Here's how the part is built. I have some questions about the finished solid (model axes, mm). A direction names the side the tool comes from. Round coordinates to 2 decimals unless told otherwise and drop trailing zeros. Order: outer loops, then holes, each group sorted by start corner. A loop starts at its lowest first (then second) coordinate and runs counter-clockwise, first axis right, second up. Notation, with made-up numbers: M -4,69.5 L 41,69.5 A20 cw 41,80.5 Z; hole C -18.5,1 d8. An arc over 180 degrees is marked long. Write item = value, one per line. Start each with the question number.
Item 1: I want a section at A-A, the plane x = 126.5. List the corners of the cut face in (y, z) for me.
Item 2: I want a section at B-B, the plane z = 3.75. State how many separate pieces and enclosed holes the cut face has, plus the area to 3 significant figures.
Item 3: I want a section at C-C, the plane x = -10. List the corners of the cut face in (y, z) for me.
Item 4: Please list where these lines run through material, in increasing order: L1, parallel to Y at x = 111, z = 3.25; L2, parallel to Y at x = 91.5, z = 6.5; L3, parallel to Y at x = 125, z = 6.
Item 5: I'm going to push flat-ended pins straight in: P1, Ø5.5, axis at x = 142.21, y = 21.4, coming from the +Z side; P2, Ø2, axis at x = -7.5, z = 6, coming from the +Y side; P3, Ø0.6, axis at y = 32.5, z = 4, coming from the +X side; P4, Ø1.4, axis at y = 17, z = 3.5, coming from the -X side. Where does each tip first touch, or does it pass through?
Item 6: For faces 1 (the face through (63.856, 15, 4)), 2 (the face through (131.856, 17, 4)), 3 (the face through (137.856, 21, 4)), 4 (the face through (134.9, 26.11, 4.37)), which set-ups out of +Z, -Z, +X, -X, +Y, -Y let a thin tool reach every point of the face, with its end or its side?
```python
from build123d import *

# Parameters (mm, degrees)
F1_DEPTH = 6.8
F2_T     = -2
F4_DEPTH = 4.8
F6_DEPTH = 4.8
F5_R     = 3.15
F7_DEPTH = 2


# Not quite as in the source:
# - a feature names something its author has since deleted; it is built from what else it names


with BuildPart() as f1:
    # F0 (on Top) → F1 (new body)
    with BuildSketch(Plane.XY):
        with BuildLine():
            Line((129.8559711718, 33.7323809788), (-4.1440288282, 33.7323809788))
            ThreePointArc((-4.1440288282, 33.7323809788), (-21.8216983579, 26.4100505084), (-29.1440288282, 8.7323809788))
            Line((-29.1440288282, 8.7323809788), (154.8559711718, 8.7323809788))
            ThreePointArc((154.8559711718, 8.7323809788), (147.5336407015, 26.4100505084), (129.8559711718, 33.7323809788))
        make_face()
    extrude(amount=F1_DEPTH)

    # F2
    f2_openings = [f1.faces().sort_by_distance(p)[0] for p in [
        (62.855971, 20.804106, 6.8),
    ]]
    offset(amount=F2_T, openings=f2_openings)

    # F3 (on face) → F4 (cut)
    with BuildSketch(Plane.XY.offset(6.8)):
        with BuildLine():
            Line((-4.1440288282, 8.7323809788), (-4.1440288282, 10.7323809788))
            Line((-4.1440288282, 10.7323809788), (-27.056907303, 10.7323809788))
            ThreePointArc((-27.056907303, 10.7323809788), (-19.6842990961, 25.6882059366), (-4.1440288282, 31.7323809788))
            Line((-4.1440288282, 31.7323809788), (-4.1440288282, 33.7323809788))
            ThreePointArc((-4.1440288282, 33.7323809788), (-21.8216983579, 26.4100505084), (-29.1440288282, 8.7323809788))
            Line((-29.1440288282, 8.7323809788), (-4.1440288282, 8.7323809788))
        make_face()
        with BuildLine():
            Line((152.7688496466, 10.7323809788), (129.8559711718, 10.7323809788))
            Line((129.8559711718, 10.7323809788), (129.8559711718, 8.7323809788))
            Line((129.8559711718, 8.7323809788), (154.8559711718, 8.7323809788))
            ThreePointArc((154.8559711718, 8.7323809788), (147.5336407015, 26.4100505084), (129.8559711718, 33.7323809788))
            Line((129.8559711718, 33.7323809788), (129.8559711718, 31.7323809788))
            ThreePointArc((129.8559711718, 31.7323809788), (145.3962414397, 25.6882059366), (152.7688496466, 10.7323809788))
        make_face()
    extrude(amount=-F4_DEPTH, mode=Mode.SUBTRACT)

    # F5 (on face) → F6 (join)
    with BuildSketch(Plane.XY.offset(2)):
        Polygon((-6.1442747528, 21.3878121691), (-6.144358997, 22.3878121656), (-6.1448644621, 28.3878121443), (-12.1442590792, 23.9015265012), (-12.1442590792, 21.4015265012), (-12.1442590792, 18.9015265012), (-6.1442747528, 14.3878121691), (-6.1442747528, 20.3878121691), align=None)
        Polygon((21.8896443518, 20.3237342556), (27.2847434124, 22.3114023306), (-6.144358997, 22.3878121656), (-6.1442747528, 21.3878121691), (-6.1442747528, 20.3878121691), align=None)
        Polygon((-4.1440288282, 10.7323809788), (1.6412445236, 10.7323809788), (16.3966900356, 16.1685977463), (27.6392464887, 20.3105922291), (21.8896443518, 20.3237342556), align=None)
        Polygon((32.9729093256, 22.2756259058), (33.0343455494, 22.298260304), (27.2847434124, 22.3114023306), (21.8896443518, 20.3237342556), (27.6392464887, 20.3105922291), align=None)
        Polygon((33.0343455494, 22.298260304), (58.6412445236, 31.7323809788), (54.8559711718, 31.7323809788), (52.8559711718, 31.7323809788), (27.2847434124, 22.3114023306), align=None)
        Polygon((61.8564633663, 20.2323809788), (61.8564633663, 22.2323807827), (33.0343455494, 22.298260304), (32.9729093256, 22.2756259058), (27.6392464887, 20.3105922291), align=None)
        Polygon((62.8559711718, 10.7323809788), (62.8559711718, 31.7323809788), (61.8564633663, 31.7323809788), (61.8564633663, 22.2323807827), (61.8564633663, 20.2323809788), (61.8564633663, 10.7323809788), align=None)
        Polygon((92.6775967943, 22.298260304), (63.8559711718, 22.2323819077), (63.8559711718, 20.2323821038), (98.0726958549, 20.3105922291), (92.7390330181, 22.2756259058), align=None)
        Polygon((72.8559711718, 31.7323809788), (67.07069782, 31.7323809788), (92.6775967943, 22.298260304), (98.4271989312, 22.3114023306), align=None)
        Polygon((98.4271989312, 22.3114023306), (92.6775967943, 22.298260304), (92.7390330181, 22.2756259058), (98.0726958549, 20.3105922291), (103.8222979918, 20.3237342556), align=None)
        Polygon((109.3152523081, 16.1685977463), (124.07069782, 10.7323809788), (129.8559711718, 10.7323809788), (103.8222979918, 20.3237342556), (98.0726958549, 20.3105922291), align=None)
        Polygon((131.8563013406, 22.3878121656), (98.4271989312, 22.3114023306), (103.8222979918, 20.3237342556), (131.8562170965, 20.3878121691), (131.8562170965, 21.3878121691), align=None)
        Polygon((131.8568068057, 28.3878121443), (131.8563013406, 22.3878121656), (131.8562170965, 21.3878121691), (131.8562170965, 20.3878121691), (131.8562170965, 14.3878121691), (137.8562014229, 18.9015265012), (137.8562014229, 21.4015265012), (137.8562014229, 23.9015265012), align=None)
        Polygon((63.8559711718, 31.7323809788), (62.8559711718, 31.7323809788), (62.8559711718, 10.7323809788), (63.8559711718, 10.7323809788), (63.8559711718, 20.2323821038), (63.8559711718, 22.2323819077), align=None)
    extrude(amount=F6_DEPTH)

    # F5 (on face) → F7 (cut)
    with BuildSketch(Plane.XY.offset(2)):
        with Locations((-16.4942590792, 21.4015265012)):
            Circle(F5_R)
        with Locations((142.2062014229, 21.4015265012)):
            Circle(F5_R)
    extrude(amount=-F7_DEPTH, mode=Mode.SUBTRACT)


solid = f1.part
```
Filled in:
q1.outline = M 8.73,0 L 33.73,0 L 33.73,6.8 L 31.73,6.8 L 31.73,2 L 22.38,2 L 22.38,6.8 L 20.38,6.8 L 20.38,2 L 11.97,2 L 11.97,6.8 L 8.73,6.8 Z
q2.separate_pieces = 1
q2.enclosed_holes = 4
q2.area = 1,180 mm^2
q3.outline = M 8.73,0 L 33.04,0 L 33.04,2 L 25.5,2 L 25.5,6.8 L 17.29,6.8 L 17.29,2 L 8.73,2 Z
q4.L1 = 8.73 to 10.73, 15.55 to 17.68, 20.34 to 22.34, 31.73 to 33.73
q4.L2 = 8.73 to 10.73, 20.3 to 22.3, 22.73 to 24.86, 31.73 to 33.73
q4.L3 = 8.73 to 12.52, 20.37 to 22.37, 31.73 to 33.73
q5.P1 = through
q5.P2 = 28.12
q5.P3 = 129.86
q5.P4 = -10.55
q6.face_1 = +Z
q6.face_2 = +Z, -Y
q6.face_3 = +Z, +X, +Y, -Y
q6.face_4 = +Z, +X, +Y
